Work out the finished part from the listing and answer in its coordinate system (mm). Face numbers are marked on the shaded views. A direction names the side the tool comes from. Give positions to 0.01 mm unless a question says otherwise; leave off trailing zeros. Write each loop counter-clockwise with the first axis right and the second up, starting at its lowest first coordinate (ties: lowest second). Pieces come first, ordered by that corner, then holes. Notation, with made-up numbers: (-6, -35.5) -> (12, -35.5) arc R21 ccw to (12, -23.5) -> close; hole circle Ø11 at (-4, 57). An arc over 180 degrees is marked (long way). Use a Markdown table: item, result. Add a question column.
Q1. Consider line 1 (X direction, y = -5, z = 8); line 2 (X direction, y = 5.5, z = 7); line 3 (Z direction, x = 0, y = 17). Determine where each line is inside the solid, lowest interval first.
Q2. For the marked faces 1, 2 and 3, determine the directions among +Z, -Z, +X, -X, +Y, -Y from which every point of the face is accessible in a straight line to the end or side of a thin tool.
Q3. Section A-A, the plane z = 3 is taken. Give the vertices of the cut face in (x, y), plus the area to 3 significant figures.
Q4. Section C-C, the plane x = -5 is taken. Give the vertices of the cut face in (y, z), plus the area to 3 significant figures.
Q5. Section B-B, the plane y = 15 is taken. Give the vertices of the cut face in (x, z).
Q6. Each of these flat-tipped pins is pushed along its axis until it touches: pin 1 Ø5 at (y, z) = (4, 4.5) entering from +X; pin 2 Ø3.5 at (x, z) = (-10, 30) entering from +Y; pin 3 Ø2 at (x, z) = (10, 32.5) entering from +Y. Where does it stop, or does it pass through?
Q7. Section D-D, the plane z = 17.5 is taken. Give the vertices of the cut face in (x, y), plus the area to 3 significant figures.
Q8. For a pull along X with two mould halves and no side action, classify the marked faces 4, 5 and 6 as pulls with the +X half, pulls with the -X half, needs draft (parallel to the pull), parting line crosses it, or undercut.
from build123d import *

# Parameters (mm, degrees)
EXTRUDE_2_DEPTH     = 50
SKETCH_2_W          = 7
SKETCH_2_H          = 35
SKETCH_2_H_2        = 5
SKETCH_2_W_2        = 6.5
CUT_EXTRUDE_1_DEPTH = 10
SKETCH_3_W          = 8
SKETCH_3_H          = 13
CUT_EXTRUDE_2_DEPTH = 5


with BuildPart() as part:
    # Эскиз1 → Бобышка-Вытянуть2 (new body)
    with BuildSketch(Plane.XY):
        Polygon((8, 20), (-8, 20), (-8, -10), (-15, -10), (-15, -20), (15, -20), (15, 0), (8, 0), (8, 10), align=None)
    extrude(amount=EXTRUDE_2_DEPTH)

    # Эскиз2 → Вырез-Вытянуть1 (cut)
    with BuildSketch(Plane(origin=(0, 0, 0), x_dir=(-1, 0, 0), z_dir=(0, 0, -1))):
        with Locations((0, 2.5)):
            Rectangle(SKETCH_2_W, SKETCH_2_H)
        with Locations((0, -17.5)):
            Rectangle(SKETCH_2_W, SKETCH_2_H_2)
        with Locations((6.75, -17.5)):
            Rectangle(SKETCH_2_W_2, SKETCH_2_H_2)
        with Locations((-6.75, -17.5)):
            Rectangle(SKETCH_2_W_2, SKETCH_2_H_2)
    extrude(amount=-CUT_EXTRUDE_1_DEPTH, mode=Mode.SUBTRACT)

    # Эскиз3 → Вырез-Вытянуть2 (cut)
    with BuildSketch(Plane.ZY.offset(8)):
        with Locations((46, 6.5)):
            Rectangle(SKETCH_3_W, SKETCH_3_H)
    extrude(amount=-CUT_EXTRUDE_2_DEPTH, mode=Mode.SUBTRACT)


solid = part.part
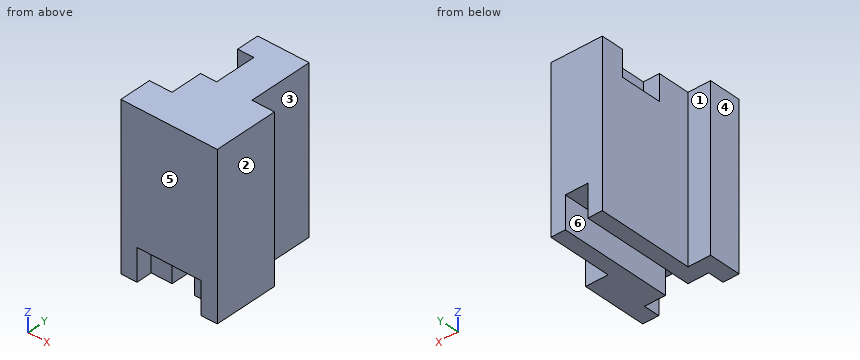
Result set:
| question | item | result |
|---|---|---|
| 1 | line 1 | x = -8 to -3.5, 3.5 to 15 |
| 1 | line 2 | x = -8 to -3.5, 3.5 to 8 |
| 1 | line 3 | z = 10 to 50 |
| 2 | face 1 | +Z, -Z, -X, +Y |
| 2 | face 2 | +Z, -Z, +X, +Y, -Y |
| 2 | face 3 | +Z, -Z, +X, +Y |
| 3 | outline | (-15, -20) -> (-10, -20) -> (-10, -15) -> (-3.5, -15) -> (-3.5, 20) -> (-8, 20) -> (-8, -10) -> (-15, -10) -> close; (3.5, -15) -> (10, -15) -> (10, -20) -> (15, -20) -> (15, 0) -> (8, 0) -> (8, 20) -> (3.5, 20) -> close |
| 3 | area | 505 mm2 |
| 4 | outline | (-20, 10) -> (-15, 10) -> (-15, 0) -> (20, 0) -> (20, 50) -> (13, 50) -> (13, 42) -> (0, 42) -> (0, 50) -> (-20, 50) -> close |
| 4 | area | 1,850 mm2 |
| 5 | outline | (-8, 0) -> (-3.5, 0) -> (-3.5, 10) -> (3.5, 10) -> (3.5, 0) -> (8, 0) -> (8, 50) -> (-8, 50) -> close |
| 6 | pin 1 | stops at x = 8 |
| 6 | pin 2 | stops at y = -10 |
| 6 | pin 3 | stops at y = 0 |
| 7 | outline | (-15, -20) -> (15, -20) -> (15, 0) -> (8, 0) -> (8, 20) -> (-8, 20) -> (-8, -10) -> (-15, -10) -> close |
| 7 | area | 850 mm2 |
| 8 | face 4 | pulls with the -X half |
| 8 | face 5 | needs draft |
| 8 | face 6 | undercut |
